```python
from build123d import *

# Parameters (mm, degrees)
SALIENTE_EXTRUIR1_DEPTH = 12.7
CROQUIS2_R              = 1.75
CORTAR_EXTRUIR1_DEPTH   = 4
CORTAR_EXTRUIR2_REACH   = 35.402
CROQUIS3_R              = 1.75


with BuildPart() as part:
    # Croquis1 → Saliente-Extruir1 (new body)
    with BuildSketch(Plane.XY):
        with BuildLine():
            Line((0, 30), (0, 42))
            Line((0, 42), (-4, 42))
            Line((-4, 42), (-4, 33.763886032))
            ThreePointArc((-4, 33.763886032), (-23.186271363, 24.867585735), (-33.401758936, 6.35))
            Line((-33.401758936, 6.35), (-33.401758936, -6.35))
            ThreePointArc((-33.401758936, -6.35), (-23.186271363, -24.867585735), (-4, -33.763886032))
            Line((-4, -33.763886032), (-4, -42))
            Line((-4, -42), (0, -42))
            Line((0, -42), (0, -30))
            ThreePointArc((0, -30), (-30, 0), (0, 30))
        make_face()
    extrude(amount=SALIENTE_EXTRUIR1_DEPTH)

    # Croquis2 → Cortar-Extruir1 (cut)
    with BuildSketch(Plane.ZY.offset(4)):
        with Locations((2.85, 37.881943016)):
            Circle(CROQUIS2_R)
        with Locations((9.85, 37.881943016)):
            Circle(CROQUIS2_R)
    cortar_extruir1 = extrude(amount=-CORTAR_EXTRUIR1_DEPTH, mode=Mode.SUBTRACT)

    # Simetría1: Cortar-Extruir1 across plane
    add(cortar_extruir1.mirror(Plane.ZX), mode=Mode.SUBTRACT)

    # Croquis3 → Cortar-Extruir2 (cut, up to next)
    with BuildSketch(Plane.ZY.offset(33.401758936), mode=Mode.PRIVATE) as cortar_extruir2_sk1:
        with Locations((2.85, 0)):
            Circle(CROQUIS3_R)
    cortar_extruir2_tool1 = extrude(cortar_extruir2_sk1.sketch, amount=-CORTAR_EXTRUIR2_REACH, mode=Mode.PRIVATE) & part.part
    add(cortar_extruir2_tool1.solids().sort_by_distance((-33.401759, 0, 2.85))[0], mode=Mode.SUBTRACT)
    # Croquis3 → Cortar-Extruir2 (cut, up to next)
    with BuildSketch(Plane.ZY.offset(33.401758936), mode=Mode.PRIVATE) as cortar_extruir2_sk2:
        with Locations((9.85, 0)):
            Circle(CROQUIS3_R)
    cortar_extruir2_tool2 = extrude(cortar_extruir2_sk2.sketch, amount=-CORTAR_EXTRUIR2_REACH, mode=Mode.PRIVATE) & part.part
    add(cortar_extruir2_tool2.solids().sort_by_distance((-33.401759, 0, 9.85))[0], mode=Mode.SUBTRACT)


solid = part.part
```
For this review, take the finished solid that the model builds, in its own axes (mm). A direction names the side the tool comes from. Give positions to 0.01 mm unless a question says otherwise; leave off trailing zeros. Loops run counter-clockwise (first coordinate to the right, second up) from the corner with the lowest first, then second, coordinate; pieces in that order, holes last. Notation, with made-up numbers: M -29,-6.75 L 17,-6.75 A29 cw 17,30.25 Z; hole C 26.25,72.5 d7. An arc over 180 degrees is marked long. One line per item, written item: value. Start each with the question number.
Q1. Add section A-A (y = 0). Give the boundary of the cut face in (x, z).
Q2. Add section D-D (x = -6.5). Give the boundary of the cut face in (y, z).
Q3. Clearance check with flat-ended pins moving along their axes: pin 1 Ø4 at (y, z) = (-23.5, 10.5) entering from -X; pin 2 Ø3 at (y, z) = (0, 9.85) entering from -X; pin 3 Ø5.5 at (y, z) = (-37.88, 9.85) entering from -X; pin 4 Ø2 at (x, z) = (-20.5, 3.5) entering from +Y. State where each tip first meets the part, or that it passes through.
Q4. For L1, parallel to Z at x = -30.75, y = 0; L2, parallel to Y at x = -2.45, z = 9.85; L3, parallel to Y at x = -4.5, z = 2.75, list the stretches that pass through material, from the lowest coordinate up.
Q5. Machinability: for faces 1 (the face through (-4, 38, 6)), 2 (the face through (-31.7, 0.526, 11.519)), 3 (the face through (-4, -38, 6)), which of the approach directions +Z, -Z, +X, -X, +Y, -Y give a long, thin tool a straight path to every point of the face, cutting with its end or side? Answer none if there is none.
Q6. Draft analysis for pull direction Z (two halves, no side actions). For faces 4 (the face through (-2.028, 39.617, 2.622)), 5 (the face through (0, 36, 6)), 6 (the face through (-30.4, 0.2, 12.7)), state which applies: released by +Z, released by -Z, zero draft, split by the parting line, or undercut.
Q7. Add section C-C (x = -22). Give the boundary of the cut face in (y, z), and give its area (3 significant figures).
Q8. Add section B-B (z = 2.85). Give the boundary of the cut face in (x, y).
Reply:
1. outline: M -33.4,0 L -30,0 L -30,1.1 L -33.4,1.1 Z; M -33.4,4.6 L -30,4.6 L -30,8.1 L -33.4,8.1 Z; M -33.4,11.6 L -30,11.6 L -30,12.7 L -33.4,12.7 Z
2. outline: M -33.37,0 L -29.29,0 L -29.29,12.7 L -33.37,12.7 Z; M 29.29,0 L 33.37,0 L 33.37,12.7 L 29.29,12.7 Z
3. pin 1: x = -26.34
3. pin 2: through
3. pin 3: x = -4
3. pin 4: y = 27.85
4. L1: 0 to 1.1, 4.6 to 8.1, 11.6 to 12.7
4. L2: -42 to -39.63, -36.13 to -29.9, 29.9 to 36.13, 39.63 to 42
4. L3: -33.7 to -29.66, 29.66 to 33.7
5. face 1: +Z, -Z, -X, +Y
5. face 2: +X, -X
5. face 3: +Z, -Z, -X, -Y
6. face 4: undercut
6. face 5: zero draft
6. face 6: released by +Z
7. outline: M -25.92,0 L -20.4,0 L -20.4,12.7 L -25.92,12.7 Z; M 20.4,0 L 25.92,0 L 25.92,12.7 L 20.4,12.7 Z
7. area: 140 mm²
8. outline: M -33.4,-6.35 A34 ccw -4,-33.76 L -4,-36.13 L 0,-36.13 L 0,-30 A30 cw -29.95,-1.75 L -33.4,-1.75 Z; M -33.4,1.75 L -29.95,1.75 A30 cw 0,30 L 0,36.13 L -4,36.13 L -4,33.76 A34 ccw -33.4,6.35 Z; M -4,-42 L 0,-42 L 0,-39.63 L -4,-39.63 Z; M -4,39.63 L 0,39.63 L 0,42 L -4,42 Z
